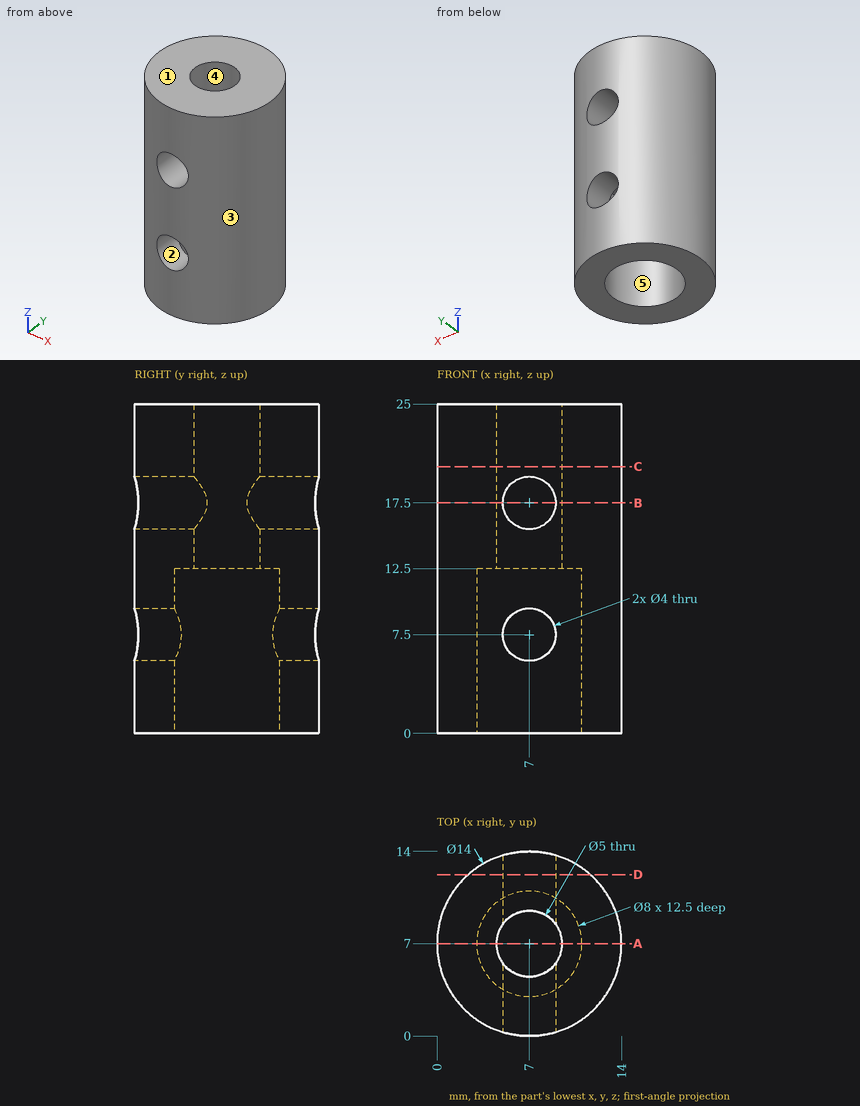
Job drawing, mm, ordinate dimensions from the low corner. One solid piece. A direction names the side the tool comes from. Round coordinates to 2 decimals unless told otherwise and drop trailing zeros. Loops run counter-clockwise (first coordinate to the right, second up) from the corner with the lowest first, then second, coordinate; pieces in that order, holes last. Notation, with made-up numbers: (50, 56) -> (82, 56) arc R21 cw to (82, 76) -> close; hole circle Ø8 at (62.25, -14). An arc over 180 degrees is marked (long way). Use a Markdown table: item, result.
1) Cut at B-B, the plane z = 17.5. List the corners of the cut face in (x, y).
The answers:
| item | result |
|---|---|
| outline | (5, 0.29) -> (5, 5.5) arc R2.5 cw to (5, 8.5) -> (5, 13.71) arc R7 ccw to start; (9, 0.29) arc R7 ccw to (9, 13.71) -> (9, 8.5) arc R2.5 cw to (9, 5.5) -> close |
2) Cut at C-C, the plane z = 20.25. List the corners of the cut face in (x, y).
The answers:
| item | result |
|---|---|
| outline | circle Ø14 at (7, 7); hole circle Ø5 at (7, 7) |
3) Probe line 1 (Y direction, x = 7, z = 4.75); line 2 (X direction, y = 6.75, z = 13); line 3 (X direction, y = 12.6, z = 7.5). List the from-to ranges inside material, lowest first. Write a range as [from, to].
The answers:
| item | result |
|---|---|
| line 1 | y = [0, 3], [11, 14] |
| line 2 | x = [0, 4.51], [9.49, 14] |
| line 3 | x = [2.8, 5], [9, 11.2] |
4) Tool access for the marked faces 4 and 5: list every direction of +Z, -Z, +X, -X, +Y, -Y with a clear straight run to the whole face (end or side of a thin tool).
The answers:
| item | result |
|---|---|
| face 4 | +Z, -Z |
| face 5 | -Z |
5) Cut at A-A, the plane y = 7. List the corners of the cut face in (x, z).
The answers:
| item | result |
|---|---|
| outline | (0, 0) -> (3, 0) -> (3, 12.5) -> (4.5, 12.5) -> (4.5, 25) -> (0, 25) -> close; (9.5, 12.5) -> (11, 12.5) -> (11, 0) -> (14, 0) -> (14, 25) -> (9.5, 25) -> close |
6) Drop flat-ended pins along their axis: pin 1 Ø1 at (x, z) = (4, 5.5) entering from -Y; pin 2 Ø6 at (y, z) = (8.5, 9) entering from -X; pin 3 Ø1.5 at (y, z) = (10, 7.5) entering from +X; pin 4 Ø4 at (y, z) = (2.5, 16) entering from -X. Give the stop position or say it passes through.
The answers:
| item | result |
|---|---|
| pin 1 | stops at y = 0.46 |
| pin 2 | stops at x = 0 |
| pin 3 | stops at x = 13.63 |
| pin 4 | stops at x = 0.46 |
7) Cut at D-D, the plane y = 12.25. List the corners of the cut face in (x, z), and give its area (3 significant figures).
The answers:
| item | result |
|---|---|
| outline | (2.37, 0) -> (11.63, 0) -> (11.63, 25) -> (2.37, 25) -> close; hole circle Ø4 at (7, 7.5); hole circle Ø4 at (7, 17.5) |
| area | 206 mm2 |
8) Pull direction X, two halves, no side cores. Call the marked faces 1, 2 and 3: pulls with the +X half, pulls with the -X half, needs draft (parallel to the pull), parting line crosses it, or undercut.
The answers:
| item | result |
|---|---|
| face 1 | needs draft |
| face 2 | undercut |
| face 3 | parting line crosses it |
